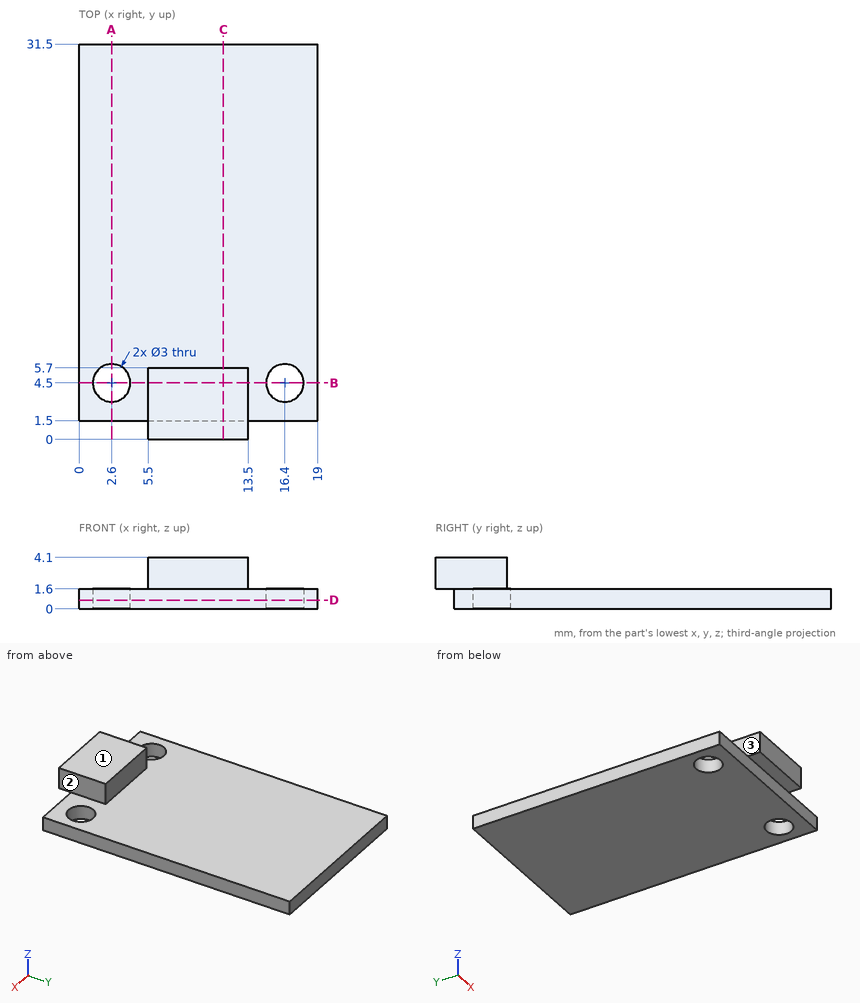
Geometry check sheet. Reference: drawing and pictorial views, mm from the part's lowest x, y, z. A direction names the side the tool comes from. Round coordinates to 2 decimals unless told otherwise and drop trailing zeros. Order: outer loops, then holes, each group sorted by start corner. A loop starts at its lowest first (then second) coordinate and runs counter-clockwise, first axis right, second up. Notation, with made-up numbers: (41.5, -0.5) - (57.5, -0.5) arc R21 cw to (57.5, 33.5) - close; hole circle Ø5 at (-28, 84). An arc over 180 degrees is marked (long way). Use a Markdown table: item, result. Add a question column.
1) Set-up check for the marked faces 1, 2 and 3: record each of +Z, -Z, +X, -X, +Y, -Y from which the full face is reachable in a straight line by a thin tool's end or side.
2) Gauge pin test, flat ends, axial feed: P1, Ø4, axis at x = 16.4, y = 4.5, coming from the +Z side; P2, Ø0.8, axis at x = 12.5, z = 1, coming from the -Y side; P3, Ø0.7, axis at x = 8, z = 3, coming from the +Y side. Record the tip position at first contact, or that the pin passes through.
3) Section check C-C (x = 11.5). Record the cut outline in (y, z).
4) Section check A-A (x = 2.6). Record the cut outline in (y, z).
5) Section check D-D (z = 0.7). Record the cut outline in (x, y).
6) Section check B-B (y = 4.5). Record the cut outline in (x, z), then the cut area to 3 significant figures.
7) Thickness scan on line 1 along Y through (x, z) = (2.6, 0.35); line 2 along Z through (x, y) = (13.5, 8); line 3 along Y through (x, z) = (12, 1.5). Record the ranges inside material, lowest first.
Established:
| question | item | result |
|---|---|---|
| 1 | face 1 | +Z, +X, -X, +Y, -Y |
| 1 | face 2 | +Z, +X, +Y, -Y |
| 1 | face 3 | +Z, -X, +Y, -Y |
| 2 | P1 | z = 1.6 |
| 2 | P2 | y = 1.5 |
| 2 | P3 | y = 5.7 |
| 3 | outline | (0, 1.6) - (1.5, 1.6) - (1.5, 0) - (31.5, 0) - (31.5, 1.6) - (5.7, 1.6) - (5.7, 4.1) - (0, 4.1) - close |
| 4 | outline | (1.5, 0) - (3, 0) - (3, 1.6) - (1.5, 1.6) - close; (6, 0) - (31.5, 0) - (31.5, 1.6) - (6, 1.6) - close |
| 5 | outline | (0, 1.5) - (19, 1.5) - (19, 31.5) - (0, 31.5) - close; hole circle Ø3 at (2.6, 4.5); hole circle Ø3 at (16.4, 4.5) |
| 6 | outline | (0, 0) - (1.1, 0) - (1.1, 1.6) - (0, 1.6) - close; (4.1, 0) - (14.9, 0) - (14.9, 1.6) - (13.5, 1.6) - (13.5, 4.1) - (5.5, 4.1) - (5.5, 1.6) - (4.1, 1.6) - close; (17.9, 0) - (19, 0) - (19, 1.6) - (17.9, 1.6) - close |
| 6 | area | 40.8 mm2 |
| 7 | line 1 | 1.5 to 3, 6 to 31.5 |
| 7 | line 2 | 0 to 1.6 |
| 7 | line 3 | 1.5 to 31.5 |
